from build123d import *

# Parameters (mm, degrees)
SKETCH2_W                   = 20
SKETCH2_H                   = 15
SHELL1_START                = -39.5000001
SHELL1_OUTLINE_R            = 85.5
SHELL1_DEPTH                = 79.0000001
SHELL1_START_2              = -235.4
SHELL1_2_OUTLINE_R          = 85.5
SHELL1_2_DEPTH              = 14.9
SHELL1_START_3              = 220.5
SHELL1_3_OUTLINE_R          = 85.5
SHELL1_3_DEPTH              = 14.9
SHELL1_START_4              = -145.650757695
SHELL1_4_OUTLINE_R          = 149.5
SHELL1_4_DEPTH              = 310.150757695
SHELL1_START_5              = -174.5
SHELL1_5_OUTLINE_R          = 39.5
SHELL1_5_DEPTH              = 89
SKETCH15_R                  = 96
CUT_EXTRUDE4_DEPTH          = 4.75
SKETCH14_R                  = 39.5
EXTRUDE2_DEPTH              = 10
F_5_8_CLEARANCE_HOLE5_D     = 16.27124
F_5_8_CLEARANCE_HOLE5_DEPTH = 20.65
F_5_8_CLEARANCE_HOLE6_D     = 16.66748
F_5_8_CLEARANCE_HOLE6_DEPTH = 20.65
SKETCH30_R                  = 96
CUT_EXTRUDE5_DEPTH          = 529.604474064


with BuildPart() as part:
    # Sketch1 → Base-Revolve (revolve)
    with BuildSketch(Plane.XY, mode=Mode.PRIVATE) as base_revolve_sk:
        Polygon((0, -185), (50, -185), (50, -175), (135, -175), (160, -150), (160, 175), (0, 175), align=None)
    revolve(base_revolve_sk.sketch.rotate(Axis((0, -64.079408138, 0), (0, 1, 0)), 90), axis=Axis((0, -64.079408138, 0), (0, 1, 0)))

    # Sketch2 → Boss-Revolve1 (revolve)
    with BuildSketch(Plane.XY, mode=Mode.PRIVATE) as boss_revolve1_sk:
        with Locations((170, 157.5)):
            Rectangle(SKETCH2_W, SKETCH2_H)
        with Locations((170, 137.5)):
            Rectangle(SKETCH2_W, SKETCH2_H)
    revolve(boss_revolve1_sk.sketch.rotate(Axis((0, 0, 0), (0, 1, 0)), 90), axis=Axis((0, 0, 0), (0, 1, 0)))

    # Sketch3 → Boss-Revolve2 (revolve)
    with BuildSketch(Plane.XY, mode=Mode.PRIVATE) as boss_revolve2_sk:
        Polygon((0, 0), (0, 52.971334051), (210, 90), (210, 139.7), (230.65, 139.7), (230.65, 96), (235.4, 96), (235.4, 0), align=None)
    boss_revolve2 = revolve(boss_revolve2_sk.sketch.rotate(Axis((0, 0, 0), (1, 0, 0)), 90), axis=Axis((0, 0, 0), (1, 0, 0)))

    # Mirror1: Boss-Revolve2 across plane
    add(boss_revolve2.mirror(Plane(origin=(0, 0, 0), x_dir=(0, 0, 1), z_dir=(1, 0, 0))))

    # Shell1: read off the stored shape, not the designer's step
    # Shell1 outline → Shell1 (cut)
    with BuildSketch(Plane.YZ.offset(SHELL1_START)):
        Circle(SHELL1_OUTLINE_R)
    extrude(amount=SHELL1_DEPTH, mode=Mode.SUBTRACT)

    # Shell1 2 outline → Shell1 2 (cut)
    with BuildSketch(Plane.YZ.offset(SHELL1_START_2)):
        Circle(SHELL1_2_OUTLINE_R)
    extrude(amount=SHELL1_2_DEPTH, mode=Mode.SUBTRACT)

    # Shell1 3 outline → Shell1 3 (cut)
    with BuildSketch(Plane.YZ.offset(SHELL1_START_3)):
        Circle(SHELL1_3_OUTLINE_R)
    extrude(amount=SHELL1_3_DEPTH, mode=Mode.SUBTRACT)

    # Shell1 4 outline → Shell1 4 (cut)
    with BuildSketch(Plane(origin=(0, 0, 0), x_dir=(1, 0, 0), z_dir=(0, 1, 0)).offset(SHELL1_START_4)):
        Circle(SHELL1_4_OUTLINE_R)
    extrude(amount=SHELL1_4_DEPTH, mode=Mode.SUBTRACT)

    # Shell1 5 outline → Shell1 5 (cut)
    with BuildSketch(Plane(origin=(0, 0, 0), x_dir=(1, 0, 0), z_dir=(0, 1, 0)).offset(SHELL1_START_5)):
        Circle(SHELL1_5_OUTLINE_R)
    extrude(amount=SHELL1_5_DEPTH, mode=Mode.SUBTRACT)

    # Shell1 6: loft between two sections, ruled curve by curve
    shell1_6_from = [
        Edge.make_three_point_arc((0, -164.5, 130.650757595), (130.650757595, -164.5, 0), (0, -164.5, -130.650757595)),
        Edge.make_three_point_arc((0, -164.5, -130.650757595), (-130.650757595, -164.5, 0), (0, -164.5, 130.650757595)),
    ]
    shell1_6_to = [
        Edge.make_three_point_arc((0, -145.650757595, 149.5), (149.5, -145.650757595, 0), (0, -145.650757595, -149.5)),
        Edge.make_three_point_arc((0, -145.650757595, -149.5), (-149.5, -145.650757595, 0), (0, -145.650757595, 149.5)),
    ]
    shell1_6 = Solid(Shell([*[Face.make_surface_from_curves(shell1_6_from[k], shell1_6_to[k]) for k in range(2)], Face(Wire(shell1_6_from)), Face(Wire(shell1_6_to))]))
    add(shell1_6, mode=Mode.SUBTRACT)

    # Shell1 7: loft between two sections, ruled curve by curve
    shell1_7_from = [
        Edge.make_three_point_arc((134.158642782, 41.530655606, 51.250412113), (134.158642782, -51.250412113, 41.530655606), (134.158642782, -41.530655606, -51.250412113)),
        Edge.make_three_point_arc((134.158642782, -41.530655606, -51.250412113), (134.158642782, 51.250412113, -41.530655606), (134.158642782, 41.530655606, 51.250412113)),
    ]
    shell1_7_to = [
        Edge.make_three_point_arc((220.5, 51.115651267, 63.078662127), (220.5, -63.078662127, 51.115651267), (220.5, -51.115651267, -63.078662127)),
        Edge.make_three_point_arc((220.5, -51.115651267, -63.078662127), (220.5, 63.078662127, -51.115651267), (220.5, 51.115651267, 63.078662127)),
    ]
    shell1_7 = Solid(Shell([*[Face.make_surface_from_curves(shell1_7_from[k], shell1_7_to[k]) for k in range(2)], Face(Wire(shell1_7_from)), Face(Wire(shell1_7_to))]))
    add(shell1_7, mode=Mode.SUBTRACT)

    # Shell1 8: loft between two sections, ruled curve by curve
    shell1_8_from = [
        Edge.make_three_point_arc((-134.158707207, 0, -65.965154404), (-134.158707207, -65.965154404, 0), (-134.158707207, 0, 65.965154404)),
        Edge.make_three_point_arc((-134.158707207, 0, 65.965154404), (-134.158707207, 65.965154404, 0), (-134.158707207, 0, -65.965154404)),
    ]
    shell1_8_to = [
        Edge.make_three_point_arc((-220.5, 0, -81.189453873), (-220.5, -81.189453873, 0), (-220.5, 0, 81.189453873)),
        Edge.make_three_point_arc((-220.5, 0, 81.189453873), (-220.5, 81.189453873, 0), (-220.5, 0, -81.189453873)),
    ]
    shell1_8 = Solid(Shell([*[Face.make_surface_from_curves(shell1_8_from[k], shell1_8_to[k]) for k in range(2)], Face(Wire(shell1_8_from)), Face(Wire(shell1_8_to))]))
    add(shell1_8, mode=Mode.SUBTRACT)

    # Sketch15 → Cut-Extrude4 (cut)
    with BuildSketch(Plane.ZY.offset(230.65)):
        Circle(SKETCH15_R)
    extrude(amount=CUT_EXTRUDE4_DEPTH, mode=Mode.SUBTRACT)

    # Sketch14 → Extrude2 (add)
    with BuildSketch(Plane(origin=(0, -174.5, 0), x_dir=(1, 0, 0), z_dir=(0, 1, 0))):
        Circle(SKETCH14_R)
    extrude(amount=EXTRUDE2_DEPTH)

    # 5/8 Clearance Hole5
    with Locations(Plane(origin=(-230.65, -86.94526051, 61.229912904), x_dir=(0, 0, 1), z_dir=(-1, 0, 0))):
        with Locations((-61.229912904, 201.24526051), (-176.596487394, 86.94526051), (-142.052217993, 167.767565599), (19.592392186, 167.767565599), (53.070087096, 86.94526051), (19.592392186, 6.12295542), (-61.229912904, -27.406492985), (-142.052217993, 6.12295542)):
            Hole(F_5_8_CLEARANCE_HOLE5_D / 2, depth=F_5_8_CLEARANCE_HOLE5_DEPTH)

    # 5/8 Clearance Hole6
    with Locations(Plane(origin=(230.65, 0, 0), x_dir=(0, 0, -1), z_dir=(1, 0, 0))):
        with Locations((-80.82230509, 80.82230509), (0, 114.3), (80.82230509, 80.82230509), (114.3, 0), (80.82230509, -80.82230509), (0, -114.351753494), (-80.82230509, -80.82230509), (-115.366574491, 0)):
            Hole(F_5_8_CLEARANCE_HOLE6_D / 2, depth=F_5_8_CLEARANCE_HOLE6_DEPTH)

    # Sketch30 → Cut-Extrude5 (cut, through all)
    with BuildSketch(Plane(origin=(230.65, 0, 0), x_dir=(0, 0, -1), z_dir=(1, 0, 0))):
        Circle(SKETCH30_R)
    extrude(amount=CUT_EXTRUDE5_DEPTH, mode=Mode.SUBTRACT)


solid = part.part
Read the model definition and answer for the solid it produces. Units are mm, in the model's axes. A direction names the side the tool comes from. Give positions to 0.01 mm unless a question says otherwise; leave off trailing zeros. Write each loop counter-clockwise with the first axis right and the second up, starting at its lowest first coordinate (ties: lowest second). Pieces come first, ordered by that corner, then holes. Notation, with made-up numbers: (5, 75.25) -> (40, 75.25) arc R13 ccw to (40, 90.25) -> close; hole circle Ø4 at (4.25, 37.5). An arc over 180 degrees is marked (long way). Answer as a JSON object with one key per item and string values. Group by question number.
1) Each of these flat-tipped pins is pushed along its axis until it touches: P1, Ø10, axis at y = 80.82, z = -80.82, coming from the +X side; P2, Ø2, axis at x = 62, y = -130.5, coming from the +Z side; P3, Ø5, axis at x = 132, z = 108, coming from the -Y side. Where does it stop, or does it pass through?
2) The mould has two halves that part along Z. Classify faces 1 (the cylindrical face through (159.69, 137.6, -83.06)), 2 (the flat face through (-1, -185, -1)), 3 (the cylindrical face through (220.18, -106.09, -1.08)): +Z half, -Z half, draft (parallel to the pull), parting line (faces both ways), or undercut.
3) Find section A-A (y = 114.3). Write down the section's boundary in (x, z), and give its area (3 significant figures).
4) A tool of negligible diameter and unlimited length cuts with its end or side. For faces 4 (the cylindrical face through (-220.18, 122.366, 1.059)), 5 (the cylindrical face through (220.18, -78.32, 88.77)), 6 (the flat face through (106, 165, -121)), 7 (the conical face through (167.52, -24.78, 78.7)), from which of +Z, -Z, +X, -X, +Y, -Y can it reach the whole face along a straight path? Write none if from no direction.
5) Consider L1, parallel to Y at x = 59, z = -107.5; L2, parallel to Y at x = -102.5, z = 137; L3, parallel to X at y = 16, z = -100.5. Determine where each line is inside the solid, lowest interval first. Write a range as from..to.
6) Find section B-B (z = 114.3). Count the separate pieces of the cut face and the enclosed holes in it, and give its area (3 significant figures).
Values follow:
{
 "1": {"P1": "stops at x = 140.89", "P2": "stops at z = 147.92", "P3": "stops at y = 130"},
 "2": {"face 1": "parting line", "face 2": "draft", "face 3": "undercut"},
 "3": {"outline": "(-230.65, -80.32) -> (-210, -80.32) -> (-210, -8.14) -> (-230.65, -8.14) -> close; (-230.65, 8.14) -> (-210, 8.14) -> (-210, 80.32) -> (-230.65, 80.32) -> close; circle Ø320 at (0, 0); (210, -80.32) -> (230.65, -80.32) -> (230.65, -8.33) -> (210, -8.33) -> close; (210, 8.33) -> (230.65, 8.33) -> (230.65, 80.32) -> (210, 80.32) -> close; hole circle Ø299 at (0, 0)", "area": "16,200 mm2"},
 "4": {"face 4": "-X", "face 5": "+X", "face 6": "+Y", "face 7": "none"},
 "5": {"L1": "y = -175..-164.5, 164.5..175", "L2": "y = 130..145, 150..165", "L3": "x = -230.65..-210, -124.5..-110.68, 110.68..124.5, 210..230.65"},
 "6": {"separate pieces": "5", "enclosed holes": "1", "area": "22,200 mm2"}
}
